from build123d import *

# Parameters (mm, degrees)
SKETCH_W                = 52.8
SKETCH_H                = 73.12
PAD_DEPTH               = 17.221
THICKNESS_T             = 1.6
SKETCH001_R             = 1.67005
PAD001_DEPTH            = 3.221
SKETCH001_MIRRORED_2_R  = 1.67005
PAD001_MIRRORED_2_DEPTH = 3.221
PAD002_DEPTH            = 1.6
SKETCH003_R             = 3.3782
POCKET_DEPTH            = 1.601
POCKET001_DEPTH         = 1.6


with BuildPart() as part:
    # Sketch → Pad (new body)
    with BuildSketch(Plane.XY):
        Rectangle(SKETCH_W, SKETCH_H)
    extrude(amount=PAD_DEPTH)

    # Thickness
    thickness_openings = [part.faces().sort_by_distance(p)[0] for p in [
        (0, 0, 17.221),
    ]]
    offset(amount=THICKNESS_T, openings=thickness_openings)

    # Sketch001 → Pad001 (join)
    with BuildSketch(Plane.XY):
        with BuildLine():
            ThreePointArc((-22.86, 28.844875), (-19.907741, 30.067741), (-18.684875, 33.02))
            Line((-18.684875, 33.02), (-18.684875, 36.56))
            Line((-26.4, 36.56), (-18.684875, 36.56))
            Line((-26.4, 28.844875), (-26.4, 36.56))
            Line((-22.86, 28.844875), (-26.4, 28.844875))
        make_face()
        with Locations((-22.86, 33.02)):
            Circle(SKETCH001_R, mode=Mode.SUBTRACT)
    pad001 = extrude(amount=PAD001_DEPTH)

    # Sketch001 Mirrored 2 → Pad001 Mirrored 2 (add)
    with BuildSketch(Plane(origin=(0, 0, 0), x_dir=(-1, 0, 0), z_dir=(0, 0, -1))):
        with BuildLine():
            ThreePointArc((-22.86, 28.844875), (-19.907741, 30.067741), (-18.684875, 33.02))
            Line((-18.684875, 33.02), (-18.684875, 36.56))
            Line((-26.4, 36.56), (-18.684875, 36.56))
            Line((-26.4, 28.844875), (-26.4, 36.56))
            Line((-22.86, 28.844875), (-26.4, 28.844875))
        make_face()
        with Locations((-22.86, 33.02)):
            Circle(SKETCH001_MIRRORED_2_R, mode=Mode.SUBTRACT)
    pad001_mirrored_2 = extrude(amount=-PAD001_MIRRORED_2_DEPTH)

    # Mirrored001: Pad001, Pad001 Mirrored 2 across XZ
    add(pad001.mirror(Plane.XZ))
    add(pad001_mirrored_2.mirror(Plane.XZ))

    # Sketch002 → Pad002 (join)
    with BuildSketch(Plane.XY):
        with BuildLine():
            Line((-47.5375, 36.16), (-47.5375, -36.16))
            ThreePointArc((-47.5375, -36.16), (-46.951714, -37.574214), (-45.5375, -38.16))
            Line((-45.5375, -38.16), (45.5375, -38.16))
            ThreePointArc((45.5375, -38.16), (46.951714, -37.574214), (47.5375, -36.16))
            Line((47.5375, -36.16), (47.5375, 36.16))
            ThreePointArc((47.5375, 36.16), (46.951714, 37.574214), (45.5375, 38.16))
            Line((45.5375, 38.16), (-45.5375, 38.16))
            ThreePointArc((-45.5375, 38.16), (-46.951714, 37.574214), (-47.5375, 36.16))
        make_face()
    extrude(amount=-PAD002_DEPTH)

    # Sketch003 → Pocket (cut, through all)
    with BuildSketch(Plane.XY):
        with Locations((-38.1, 25.4)):
            Circle(SKETCH003_R)
        with Locations((38.1, 25.4)):
            Circle(SKETCH003_R)
        with Locations((-38.1, -25.4)):
            Circle(SKETCH003_R)
        with Locations((38.1, -25.4)):
            Circle(SKETCH003_R)
    extrude(amount=-POCKET_DEPTH, mode=Mode.SUBTRACT)

    # Sketch004 (on DatumPlane) → Pocket001 (cut)
    with BuildSketch(Plane.YZ.offset(28)):
        with BuildLine():
            Line((-6, 17.221), (6, 17.221))
            Line((6, 17.221), (6, 16.221))
            ThreePointArc((4, 14.221), (5.414214, 14.806786), (6, 16.221))
            Line((-4, 14.221), (4, 14.221))
            ThreePointArc((-6, 16.221), (-5.414214, 14.806786), (-4, 14.221))
            Line((-6, 17.221), (-6, 16.221))
        make_face()
    extrude(amount=-POCKET001_DEPTH, mode=Mode.SUBTRACT)


solid = part.part
Source: CAD feature listing. Evaluate the final solid. Frame: model axes, mm. A direction names the side the tool comes from. Round coordinates to 2 decimals unless told otherwise and drop trailing zeros. Loops run counter-clockwise (first coordinate to the right, second up) from the corner with the lowest first, then second, coordinate; pieces in that order, holes last. Notation, with made-up numbers: (88.5, 40.25) - (96.5, 40.25) arc R25 cw to (96.5, 53.25) - close; hole circle Ø9 at (85.5, -17.5). An arc over 180 degrees is marked (long way). Write item = value, one per line. Start each with the question number.
(1) Section query B-B, the plane z = 9.5. Output: boundary loops of the cut face in (x, y), plus the area to 3 significant figures.
(2) Section query C-C, the plane y = -15. Output: boundary loops of the cut face in (x, z), plus the area to 3 significant figures.
(3) Section query D-D, the plane y = 27. Output: boundary loops of the cut face in (x, z).
(4) Section query A-A, the plane x = 38.1. Output: boundary loops of the cut face in (y, z), plus the area to 3 significant figures.
(5) Set-up query: faces 1 (the face through (24.3, -31.9, 3.221)), 2 (the face through (-40.781, -27.456, -0.789)), 3 (the face through (27.21, -5.43, 14.82)). Return all of +Z, -Z, +X, -X, +Y, -Y with unobstructed straight access to the full face (end or side cutting, diameter ignored); none if empty.
(6) Ray query, line 1 along Y through (x, z) = (-22.86, 1.15); line 2 along Y through (x, z) = (-38.1, -0.4); line 3 along X through (y, z) = (-33.02, 0.7). Return the intervals inside material, ascending. Write a range as from..to.
(7) Pull-direction query (Y, two-part tool) for faces 4 (the face through (-46.967, -37.559, -0.789)), 5 (the face through (-1, 1, -1.6)), 6 (the face through (0, 1, 0)), 7 (the face through (46.967, 37.559, -0.789)); classes: +Y half, -Y half, draft (parallel to the pull), parting line (faces both ways), or undercut.
(8) Pin query (flat end, axial travel): pin 1 (5.5 mm diameter, centred on x = 38.1, y = -25.4, fed in from +Z); pin 2 (6 mm diameter, centred on x = -21, y = -31, fed in from +Z); pin 3 (1.5 mm diameter, centred on x = 18, y = 10, fed in from +Z); pin 4 (10 mm diameter, centred on y = -7, z = 6, fed in from -X). Return the tip coordinate at first contact, or that it passes through.
Conclusion:
q1.outline = (-28, -36.56) arc R1.6 ccw to (-26.4, -38.16) - (26.4, -38.16) arc R1.6 ccw to (28, -36.56) - (28, 36.56) arc R1.6 ccw to (26.4, 38.16) - (-26.4, 38.16) arc R1.6 ccw to (-28, 36.56) - close; hole (-26.4, -36.56) - (26.4, -36.56) - (26.4, 36.56) - (-26.4, 36.56) - close
q1.area = 411 mm2
q2.outline = (-47.54, -1.6) - (47.54, -1.6) - (47.54, 0) - (28, 0) - (28, 17.22) - (26.4, 17.22) - (26.4, 0) - (-26.4, 0) - (-26.4, 17.22) - (-28, 17.22) - (-28, 0) - (-47.54, 0) - close
q2.area = 207 mm2
q3.outline = (-47.54, -1.6) - (-41.08, -1.6) - (-41.08, 0) - (-47.54, 0) - close; (-35.12, -1.6) - (35.12, -1.6) - (35.12, 0) - (28, 0) - (28, 17.22) - (26.4, 17.22) - (26.4, 0) - (-26.4, 0) - (-26.4, 17.22) - (-28, 17.22) - (-28, 0) - (-35.12, 0) - close; (41.08, -1.6) - (47.54, -1.6) - (47.54, 0) - (41.08, 0) - close
q4.outline = (-38.16, -1.6) - (-28.78, -1.6) - (-28.78, 0) - (-38.16, 0) - close; (-22.02, -1.6) - (22.02, -1.6) - (22.02, 0) - (-22.02, 0) - close; (28.78, -1.6) - (38.16, -1.6) - (38.16, 0) - (28.78, 0) - close
q4.area = 100 mm2
q5.face_1 = +Z
q5.face_2 = +Z, -Z
q5.face_3 = +Z, +X
q6.line_1 = -38.16..-34.69, -31.35..-28.84, 28.84..31.35, 34.69..38.16
q6.line_2 = -38.16..-28.78, -22.02..22.02, 28.78..38.16
q6.line_3 = -28..-24.53, -21.19..-18.68, 18.68..21.19, 24.53..28
q7.face_4 = -Y half
q7.face_5 = draft
q7.face_6 = undercut
q7.face_7 = +Y half
q8.pin_1 = through
q8.pin_2 = 3.22
q8.pin_3 = 0
q8.pin_4 = -28
